Geometry check sheet. Reference: the model listing, model coordinates, mm. Face numbers are marked on the shaded views. A direction names the side the tool comes from. Coordinates: 2 decimals unless noted, no trailing zeros. Order: outer loops, then holes, each group sorted by start corner. A loop starts at its lowest first (then second) coordinate and runs counter-clockwise, first axis right, second up. Notation, with made-up numbers: M 68.25,72.5 L 103.25,72.5 A30 ccw 103.25,98.5 Z; hole C -38,7.25 d10. An arc over 180 degrees is marked long. One line per item, written item: value. Start each with the question number.
1) Thickness scan on L1, parallel to Y at x = 0, z = 4.7; L2, parallel to Z at x = -7.25, y = 1.5; L3, parallel to X at y = 7.75, z = 1.5. Record the ranges inside material, lowest first. Write a range as from..to.
2) Sectioned sample at D-D, the plane z = 2. Enter the section's corners in (x, y).
3) Go/stop test with flat-tipped pins: P1, Ø1.5, axis at x = 2, z = 1.5, coming from the +Y side; P2, Ø1, axis at x = -1.5, y = -1.5, coming from the -Z side; P3, Ø1.9, axis at y = 1.5, z = 1, coming from the -X side; P4, Ø6, axis at x = 4, y = -2.5, coming from the -Z side. Record where each tip stops, or that it passes through.
4) Access from +Z, -Z, +X, -X, +Y, -Y to the whole of each face (thin tool, end or side, straight path). Record for the marked faces 4, 5 and 6.
5) Sectioned sample at A-A, the plane y = 0. Enter the section's corners in (x, z), then the cut area to 4 significant figures.
6) Draft check along X on the marked faces 1, 2 and 3. Enter one of: pulls with the +X half, pulls with the -X half, needs draft (parallel to the pull), parting line crosses it, or undercut.
7) Sectioned sample at C-C, the plane z = 5.75. Enter the section's corners in (x, y).
```python
from build123d import *

# Parameters (mm, degrees)
SKETCH_R        = 11.45
PAD_DEPTH       = 7.7
SKETCH003_R     = 7.95
POCKET_DEPTH    = 5
POCKET001_DEPTH = 1.7


with BuildPart() as part:
    # Sketch → Pad (new body)
    with BuildSketch(Plane.XY):
        Circle(SKETCH_R)
    extrude(amount=PAD_DEPTH)

    # Sketch003 (on Face3 of Pad) → Pocket (cut)
    with BuildSketch(Plane.XY.offset(7.7)):
        Circle(SKETCH003_R)
    extrude(amount=-POCKET_DEPTH, mode=Mode.SUBTRACT)

    # Sketch002 → Pocket001 (cut)
    with BuildSketch(Plane(origin=(0, 0, 0), x_dir=(1, 0, 0), z_dir=(0, 0, -1))):
        Polygon((-9.7, 5.1), (-5, 5.1), (-5, 9.7), (5, 9.7), (5, 5.1), (9.7, 5.1), (9.7, -5.1), (5, -5.1), (5, -9.7), (-5, -9.7), (-5, -5.1), (-9.7, -5.1), align=None)
    extrude(amount=-POCKET001_DEPTH, mode=Mode.SUBTRACT)


solid = part.part
```
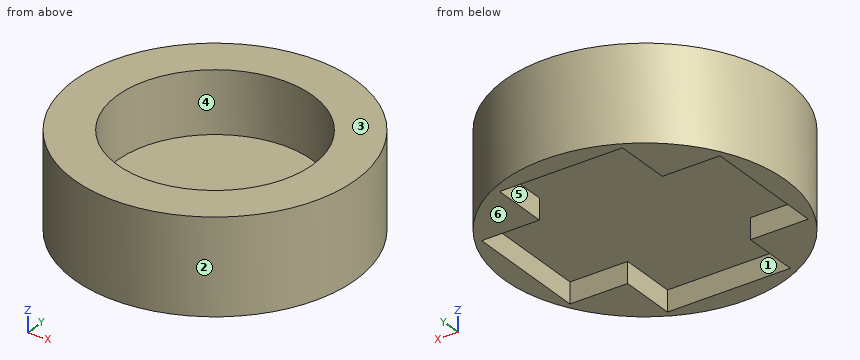
Final values:
1. L1: y = -11.45..-7.95, 7.95..11.45
1. L2: z = 1.7..2.7
1. L3: x = -8.43..-5, 5..8.43
2. outline: C 0,0 d22.9
3. P1: stops at y = 11.38
3. P2: stops at z = 1.7
3. P3: stops at x = -11.44
3. P4: stops at z = 0
4. face 4: +Z
4. face 5: -Z
4. face 6: -Z, +X, -X, +Y, -Y
5. outline: M -11.45,0 L -9.7,0 L -9.7,1.7 L 9.7,1.7 L 9.7,0 L 11.45,0 L 11.45,7.7 L 7.95,7.7 L 7.95,2.7 L -7.95,2.7 L -7.95,7.7 L -11.45,7.7 Z
5. area: 63.85 mm^2
6. face 1: undercut
6. face 2: parting line crosses it
6. face 3: needs draft
7. outline: C 0,0 d22.9; hole C 0,0 d15.9
